Part model, mm, in its own coordinate system. A direction names the side the tool comes from. Round coordinates to 2 decimals unless told otherwise and drop trailing zeros. Order: outer loops, then holes, each group sorted by start corner. A loop starts at its lowest first (then second) coordinate and runs counter-clockwise, first axis right, second up. Notation, with made-up numbers: (-30, 50) -> (5, 50) arc R18 cw to (5, 76) -> close; hole circle Ø1 at (75, -13.75). An arc over 180 degrees is marked (long way). Return JSON: item names as keys, results as strings. Group by question number.
from build123d import *

# Parameters (mm, degrees)
F0_R            = 8
F1_DEPTH        = 20
F2_R            = 5
F3_DEPTH        = 20
F5_DEPTH        = 16
F5_COPIES_COUNT = 3
F6_SIZE         = 0.49999
F7_R            = 0.5
F9_D            = 4
F9_DEPTH        = 14
F9_TIP          = 1.2017212381
F10_R           = 2.1
F11_DEPTH       = 8.25
F12_SIZE        = 3


# Not quite as in the source:
# - a fillet or chamfer is up to 0.001 mm smaller than in the source, because OpenCascade refuses the exact size
# - a pattern or mirror of a feature is missing from the dataset's text; its kind, count and spacing are read off the source's solid


with BuildPart() as f1:
    # F0 (on Front) → F1 (new body)
    with BuildSketch(Plane.XZ):
        Circle(F0_R)
    extrude(amount=-F1_DEPTH)

    # F2 (on face) → F3 (join)
    with BuildSketch(Plane(origin=(0, 20, 0), x_dir=(-1, 0, 0), z_dir=(0, 1, 0))):
        Circle(F2_R)
    extrude(amount=F3_DEPTH)

    # F4 (on face) → F5 (cut)
    with BuildSketch(Plane(origin=(0, 40, 0), x_dir=(-1, 0, 0), z_dir=(0, 1, 0))):
        with BuildLine():
            ThreePointArc((2.1794494718, 4.5), (0, 5), (-2.1794494718, 4.5))
            Line((-2.1794494718, 4.5), (2.1794494718, 4.5))
        make_face()
    f5 = extrude(amount=-F5_DEPTH, mode=Mode.SUBTRACT)

    # F5_copies: F5 ×3 about axis
    f5_copies_axis = Axis((0, 0, 0), (0, 1, 0))
    for i in range(1, F5_COPIES_COUNT):
        add(f5.rotate(f5_copies_axis, i * 360 / F5_COPIES_COUNT), mode=Mode.SUBTRACT)

    # F6 (size 0.5 in the source; OpenCascade refuses exactly that, so slightly less here)
    f6_edges = [f1.edges().sort_by_distance(p)[0] for p in [
        (4.330127, 40, 2.5),
        (-4.996709, 40, -0.18139),
        (0, 40, -5),
        (-4.236582, 40, 2.655443),
    ]]
    chamfer(f6_edges, length=F6_SIZE)

    # F7
    f7_edges = [f1.edges().sort_by_distance(p)[0] for p in [
        (-8, 20, 0),
        (5, 20, 0),
    ]]
    fillet(f7_edges, radius=F7_R)

    # F9
    with Locations(Plane.XZ):
        with Locations((0, 0)):
            Hole(F9_D / 2, depth=F9_DEPTH)
            with Locations((0, 0, -(F9_DEPTH + F9_TIP / 2))):  # 118° drill point
                Cone(0, F9_D / 2, F9_TIP, mode=Mode.SUBTRACT)

    # F10 (on Right) → F11 (cut, symmetric)
    with BuildSketch(Plane.YZ):
        with Locations((10, 0)):
            Circle(F10_R)
    extrude(amount=F11_DEPTH, both=True, mode=Mode.SUBTRACT)

    # F12
    f12_edges = [f1.edges().sort_by_distance(p)[0] for p in [
        (-8, 0, 0),
    ]]
    chamfer(f12_edges, length=F12_SIZE)


solid = f1.part
(1) Tool access for faces 4 (the flat face through (4.1, 24, -2.4)), 5 (the flat face through (-3.912, 32.112, -2.224)), 6 (the flat face through (0, 32, 4.5)), 7 (the cylindrical face through (-2.307, 29.867, -4.436)), 8 (the cylindrical face through (-0.923, 12.717, -1.774)): list every direction of +Z, -Z, +X, -X, +Y, -Y with a clear straight run to the whole face (end or side of a thin tool).
(2) Pin check, flat tips, straight feed: P1, Ø1, axis at y = 23.5, z = 3, coming from the -X side; P2, Ø8, axis at y = 28.5, z = -0.5, coming from the -X side; P3, Ø6, axis at y = 21.5, z = 5, coming from the +X side. Stop position of each tip, or through.
(3) Probe L1, parallel to X at y = 7, z = 0; L2, parallel to Y at x = 3, z = 0. List the from-to ranges inside material, lowest first. Write a range as [from, to].
(4) Saw through at A-A, the plane y = 33. List the corners of the cut face in (x, z).
(5) Mould opens along X. For faces 1 (the flat face through (-4, 20, 4)), 2 (the conical face through (-0.08, 14.99, -0.34)), 3 (the conical face through (3.98, 39.86, 2.38)) say: pulls with the +X half, pulls with the -X half, needs draft (parallel to the pull), parting line crosses it, or undercut.
(6) Saw through at C-C, the plane y = 22.5. List the corners of the cut face in (x, z).
(7) Saw through at B-B, the plane y = 10. List the corners of the cut face in (x, z).
(8) Saw through at D-D, the plane y = 16.5. List the corners of the cut face in (x, z), and give its area (3 significant figures).
Results are:
{
 "1": {"face 4": "-Z, +X, +Y", "face 5": "-Z, -X, +Y", "face 6": "+Z, +X, -X, +Y", "face 7": "+Y", "face 8": "-Y"},
 "2": {"P1": "stops at x = -4.33", "P2": "stops at x = -5", "P3": "stops at x = 7.53"},
 "3": {"L1": "x = [-8, -2], [2, 8]", "L2": "y = [0, 7.9], [12.1, 40]"},
 "4": {"outline": "(-4.99, -0.36) -> (-2.81, -4.14) arc R5 ccw to (2.81, -4.14) -> (4.99, -0.36) arc R5 ccw to (2.18, 4.5) -> (-2.18, 4.5) arc R5 ccw to start"},
 "5": {"face 1": "needs draft", "face 2": "undercut", "face 3": "pulls with the +X half"},
 "6": {"outline": "circle Ø10 at (0, 0)"},
 "7": {"outline": "(-7.72, -2.1) arc R8 ccw to (7.72, -2.1) -> close; (-7.72, 2.1) -> (7.72, 2.1) arc R8 ccw to start"},
 "8": {"outline": "circle Ø16 at (0, 0)", "area": "201 mm^2"}
}
